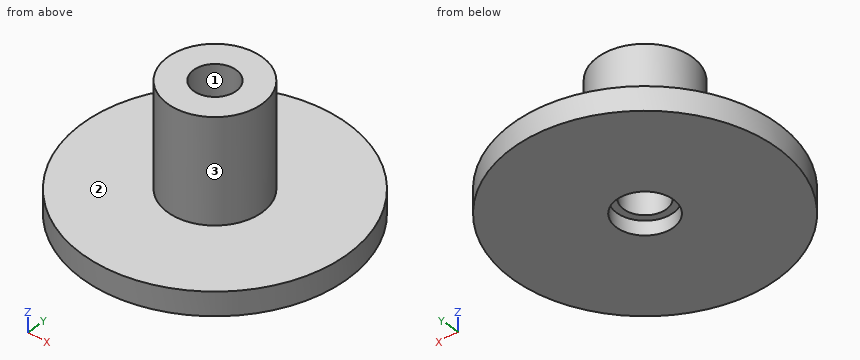
from build123d import *

# Parameters (mm, degrees)
F0_R     = 28
F1_DEPTH = 5
F2_R     = 10
F3_DEPTH = 22
F4_R     = 6
F5_DEPTH = 3
F6_R     = 4.5
F7_DEPTH = 27


with BuildPart() as f1:
    # F0 (on Top) → F1 (new body)
    with BuildSketch(Plane.XY):
        Circle(F0_R)
    extrude(amount=F1_DEPTH)

    # F2 (on face) → F3 (join)
    with BuildSketch(Plane.XY.offset(5)):
        Circle(F2_R)
    extrude(amount=F3_DEPTH)

    # F4 (on face) → F5 (cut)
    with BuildSketch(Plane(origin=(0, 0, 0), x_dir=(1, 0, 0), z_dir=(0, 0, -1))):
        Circle(F4_R)
    extrude(amount=-F5_DEPTH, mode=Mode.SUBTRACT)

    # F6 (on face) → F7 (cut)
    with BuildSketch(Plane(origin=(0, 0, 0), x_dir=(1, 0, 0), z_dir=(0, 0, -1))):
        Circle(F6_R)
    extrude(amount=-F7_DEPTH, mode=Mode.SUBTRACT)


solid = f1.part
Design review of the part built by this model. Coordinates are the model's own, in mm. Face numbers are marked on the shaded views. Give positions to 0.01 mm unless a question says otherwise; leave off trailing zeros. Order: outer loops, then holes, each group sorted by start corner. A loop starts at its lowest first (then second) coordinate and runs counter-clockwise, first axis right, second up. Notation, with made-up numbers: (15.5, 42.25) - (20.5, 42.25) arc R12 cw to (20.5, 55.25) - close; hole circle Ø1 at (15.5, -29.75). An arc over 180 degrees is marked (long way). Write item = value, one per line. Start each with the question number.
Q1. Mouldability with a two-part tool opening along Y and no side actions: class the marked faces 1, 2 and 3 as released by +Y, released by -Y, zero draft, split by the parting line, or undercut.
Q2. We need section A-A on x = 0. State the section outline as (y, z) points, plus the area to 3 significant figures.
Q3. We need section C-C on z = 19. State the section outline as (x, y) points.
Q4. We need section D-D on x = -8. State the section outline as (y, z) points, plus the area to 3 significant figures.
Q5. To check wall thickness, follow L1, parallel to Y at x = 0, z = 0.9; L2, parallel to Y at x = 0, z = 15.5; L3, parallel to Z at x = 18.5, y = 2. State the ranges of each line that lie inside material, in increasing order. Write a range as from..to.
Q6. Clearance check with flat-ended pins moving along their axes: pin 1 Ø6 at (y, z) = (7.5, 22) entering from +X; pin 2 Ø1.5 at (y, z) = (-1.5, 18) entering from -X; pin 3 Ø12 at (x, z) = (9.5, 23) entering from +Y; pin 4 Ø6 at (x, y) = (3, 1.5) entering from -Z. State where each tip first meets the part, or that it passes through.
Working result:
q1.face_1 = undercut
q1.face_2 = zero draft
q1.face_3 = split by the parting line
q2.outline = (-28, 0) - (-6, 0) - (-6, 3) - (-4.5, 3) - (-4.5, 27) - (-10, 27) - (-10, 5) - (-28, 5) - close; (4.5, 3) - (6, 3) - (6, 0) - (28, 0) - (28, 5) - (10, 5) - (10, 27) - (4.5, 27) - close
q2.area = 468 mm²
q3.outline = circle Ø20 at (0, 0); hole circle Ø9 at (0, 0)
q4.outline = (-26.83, 0) - (26.83, 0) - (26.83, 5) - (6, 5) - (6, 27) - (-6, 27) - (-6, 5) - (-26.83, 5) - close
q4.area = 532 mm²
q5.L1 = -28..-6, 6..28
q5.L2 = -10..-4.5, 4.5..10
q5.L3 = 0..5
q6.pin_1 = 8.93
q6.pin_2 = -9.97
q6.pin_3 = 9.37
q6.pin_4 = 0
